Input: part model. Units: mm. Frame: model coordinates. Round coordinates to 2 decimals unless told otherwise and drop trailing zeros. Loops run counter-clockwise (first coordinate to the right, second up) from the corner with the lowest first, then second, coordinate; pieces in that order, holes last. Notation, with made-up numbers: (70.5, 3) -> (104.5, 3) arc R24 cw to (104.5, 40) -> close; hole circle Ø8 at (3, -1). An arc over 180 degrees is marked (long way). Answer as a JSON object with one key per item and string values.
```python
from build123d import *

# Parameters (mm, degrees)
SKETCH1_R                                           = 3.75
BOSS_EXTRUDE1_DEPTH                                 = 5
CSK_FOR_M3_COUNTERSUNK_FLAT_HEAD_SCREW1_D           = 3.4
CSK_FOR_M3_COUNTERSUNK_FLAT_HEAD_SCREW1_CSINK_D     = 6.3
CSK_FOR_M3_COUNTERSUNK_FLAT_HEAD_SCREW1_CSINK_ANGLE = 90
M3_CLEARANCE_HOLE3_D                                = 3.4
M3_CLEARANCE_HOLE3_DEPTH                            = 5
M3_CLEARANCE_HOLE3_TIP                              = 1.021463052


with BuildPart() as part:
    # Sketch1 → Boss-Extrude1 (new body)
    with BuildSketch(Plane(origin=(0, 0, 0), x_dir=(0, 0, -1), z_dir=(1, 0, 0))):
        with BuildLine():
            Line((-30, -13.75), (30, -13.75))
            ThreePointArc((30, -13.75), (33.535533906, -12.285533906), (35, -8.75))
            Line((35, -8.75), (35, 8.75))
            ThreePointArc((35, 8.75), (33.535533906, 12.285533906), (30, 13.75))
            Line((30, 13.75), (-30, 13.75))
            ThreePointArc((-30, 13.75), (-33.535533906, 12.285533906), (-35, 8.75))
            Line((-35, 8.75), (-35, -8.75))
            ThreePointArc((-35, -8.75), (-33.535533906, -12.285533906), (-30, -13.75))
        make_face()
        Circle(SKETCH1_R, mode=Mode.SUBTRACT)
    extrude(amount=BOSS_EXTRUDE1_DEPTH)

    # CSK for M3 Countersunk Flat Head Screw1 (through all)
    with Locations(Plane(origin=(5, 0, 10), x_dir=(0, 0, 1), z_dir=(1, 0, 0))):
        with Locations((0, 0), (-20, 0)):
            CounterSinkHole(CSK_FOR_M3_COUNTERSUNK_FLAT_HEAD_SCREW1_D / 2, CSK_FOR_M3_COUNTERSUNK_FLAT_HEAD_SCREW1_CSINK_D / 2, counter_sink_angle=CSK_FOR_M3_COUNTERSUNK_FLAT_HEAD_SCREW1_CSINK_ANGLE)

    # M3 Clearance Hole3
    with Locations(Plane(origin=(0, 8, 30), x_dir=(0, 0, -1), z_dir=(-1, 0, 0))):
        with Locations((0, 0), (0, 16), (60, 16), (60, 0)):
            Hole(M3_CLEARANCE_HOLE3_D / 2, depth=M3_CLEARANCE_HOLE3_DEPTH)
            with Locations((0, 0, -(M3_CLEARANCE_HOLE3_DEPTH + M3_CLEARANCE_HOLE3_TIP / 2))):  # 118° drill point
                Cone(0, M3_CLEARANCE_HOLE3_D / 2, M3_CLEARANCE_HOLE3_TIP, mode=Mode.SUBTRACT)


solid = part.part
```
1) Contact query for a flat-ended pin moving along its axis: P1, Ø3, axis at y = 0, z = 10, coming from the -X side. Output: stop coordinate, or through.
Output:
{"P1": "passes through"}
2) Section D-D, the plane y = 8. Output: boundary loops of the cut face in (x, z).
Output:
{"outline": "(0, -35) -> (5, -35) -> (5, -31.7) -> (0, -31.7) -> close; (0, -28.3) -> (5, -28.3) -> (5, 28.3) -> (0, 28.3) -> close; (0, 31.7) -> (5, 31.7) -> (5, 35) -> (0, 35) -> close"}
3) Section C-C, the plane z = -10. Output: boundary loops of the cut face in (x, y), plus the area to 3 significant figures.
Output:
{"outline": "(0, -13.75) -> (5, -13.75) -> (5, -3.15) -> (3.55, -1.7) -> (0, -1.7) -> close; (0, 1.7) -> (3.55, 1.7) -> (5, 3.15) -> (5, 13.75) -> (0, 13.75) -> close", "area": "118 mm^2"}
4) Section B-B, the plane y = 0. Output: boundary loops of the cut face in (x, z).
Output:
{"outline": "(0, -35) -> (5, -35) -> (5, -13.15) -> (3.55, -11.7) -> (0, -11.7) -> close; (0, -8.3) -> (3.55, -8.3) -> (5, -6.85) -> (5, -3.75) -> (0, -3.75) -> close; (0, 3.75) -> (5, 3.75) -> (5, 6.85) -> (3.55, 8.3) -> (0, 8.3) -> close; (0, 11.7) -> (3.55, 11.7) -> (5, 13.15) -> (5, 35) -> (0, 35) -> close"}
5) Section A-A, the plane x = 1.6. Output: boundary loops of the cut face in (y, z).
Output:
{"outline": "(-13.75, -30) arc R5 ccw to (-8.75, -35) -> (8.75, -35) arc R5 ccw to (13.75, -30) -> (13.75, 30) arc R5 ccw to (8.75, 35) -> (-8.75, 35) arc R5 ccw to (-13.75, 30) -> close; hole circle Ø3.4 at (-8, -30); hole circle Ø3.4 at (-8, 30); hole circle Ø7.5 at (0, 0); hole circle Ø3.4 at (0, -10); hole circle Ø3.4 at (0, 10); hole circle Ø3.4 at (8, -30); hole circle Ø3.4 at (8, 30)"}
6) Ray query, probe 1 along Z at (x, y) = (3.5, -8); probe 2 along Y at (x, z) = (3.15, 30); probe 3 along Y at (x, z) = (3.45, 0). Return the intervals inside material, ascending.
Output:
{"probe 1": "z = -35 to -31.7, -28.3 to 28.3, 31.7 to 35", "probe 2": "y = -13.75 to -9.7, -6.3 to 6.3, 9.7 to 13.75", "probe 3": "y = -13.75 to -3.75, 3.75 to 13.75"}
7) Draft query along Y for faces 1 (the face through (2.54, 8.65, -28.43)), 2 (the face through (2.54, -7.35, 31.57)), 3 (the face through (2.46, 12.25, -33.57)), 4 (the face through (0, 6, 0)). Return one class per face: +Y half, -Y half, draft (parallel to the pull), parting line (faces both ways), or undercut.
Output:
{"face 1": "undercut", "face 2": "undercut", "face 3": "+Y half", "face 4": "draft"}
